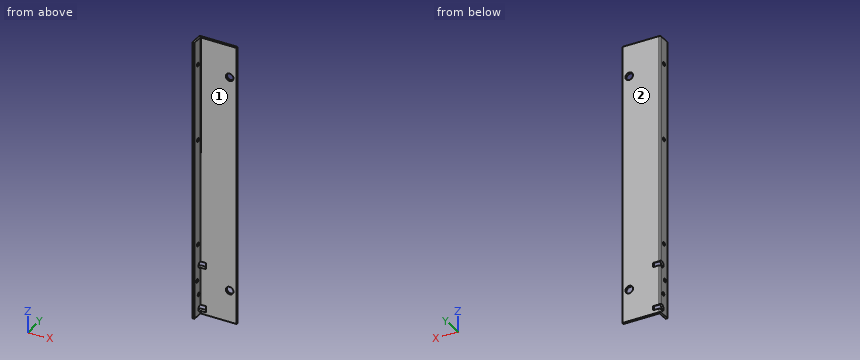
```python
from build123d import *

# Parameters (mm, degrees)
EXTRUDE_1_DEPTH     = 1100
SKETCH_2_R          = 15
CUT_EXTRUDE_1_DEPTH = 10
SKETCH_3_R          = 7
CUT_EXTRUDE_2_DEPTH = 10
SKETCH_4_R          = 12.5
CUT_EXTRUDE_3_DEPTH = 30
SKETCH_5_R          = 7
CUT_EXTRUDE_4_DEPTH = 10


with BuildPart() as part:
    # 草图1 → 凸台-拉伸1 (new body)
    with BuildSketch(Plane.XY):
        with BuildLine():
            Line((0, 0), (0, 45))
            ThreePointArc((0, 45), (1.464466094, 48.535533906), (5, 50))
            Line((5, 50), (150, 50))
            Line((150, 50), (150, 42))
            Line((150, 42), (10, 42))
            ThreePointArc((10, 42), (8.585786438, 41.414213562), (8, 40))
            Line((8, 40), (8, 0))
            Line((8, 0), (0, 0))
        make_face()
    extrude(amount=EXTRUDE_1_DEPTH)

    # 草图2 → 切除-拉伸1 (cut)
    with BuildSketch(Plane(origin=(0, 50, 0), x_dir=(1, 0, 0), z_dir=(0, 1, 0))):
        with Locations(Location((123, -975, 0), (0, 0, 270))):
            Circle(SKETCH_2_R)
        with Locations(Location((123, -125, 0), (0, 0, 270))):
            Circle(SKETCH_2_R)
    extrude(amount=-CUT_EXTRUDE_1_DEPTH, mode=Mode.SUBTRACT)

    # 草图3 → 切除-拉伸2 (cut)
    with BuildSketch(Plane.ZY):
        with Locations((283.54329503, 25.022549618)):
            Circle(SKETCH_3_R)
        with Locations((140.939449508, 19.704656779)):
            Circle(SKETCH_3_R)
        with Locations(Location((22.762519147, 40.542438099, 0), (0, 0, 355.555628173))):
            Circle(SKETCH_3_R)
        with Locations(Location((194.910597259, 40.650885608, 0), (0, 0, 354.6647218))):
            Circle(SKETCH_3_R)
        with Locations((81.850984328, 30.123547439)):
            Circle(SKETCH_3_R)
    extrude(amount=-CUT_EXTRUDE_2_DEPTH, mode=Mode.SUBTRACT)

    # 草图4 → 切除-拉伸3 (cut)
    with BuildSketch(Plane.ZY):
        with Locations((22.762519147, 40.542438099)):
            Circle(SKETCH_4_R)
        with Locations((194.910597259, 40.650885608)):
            Circle(SKETCH_4_R)
    extrude(amount=-CUT_EXTRUDE_3_DEPTH, mode=Mode.SUBTRACT)

    # 草图5 → 切除-拉伸4 (cut)
    with BuildSketch(Plane.ZY):
        with Locations((1000, 25.022549618)):
            Circle(SKETCH_5_R)
        with Locations((700, 25.022549618)):
            Circle(SKETCH_5_R)
    extrude(amount=-CUT_EXTRUDE_4_DEPTH, mode=Mode.SUBTRACT)


solid = part.part
```
Part model, mm, in its own coordinate system. Face numbers are marked on the shaded views. A direction names the side the tool comes from. Round coordinates to 2 decimals unless told otherwise and drop trailing zeros. Order: outer loops, then holes, each group sorted by start corner. A loop starts at its lowest first (then second) coordinate and runs counter-clockwise, first axis right, second up. Notation, with made-up numbers: M 68.5,-31 L 84.5,-31 A23 ccw 84.5,7 Z; hole C 83.25,-9 d7. An arc over 180 degrees is marked long. Answer in a Markdown table with one row per item. Add a question column.
Q1. Cut at D-D on x = 82.5. Give the cut face in (y, z), and give its area (3 significant figures).
Q2. Cut at B-B on x = 123. Give the cut face in (y, z), and give its area (3 significant figures).
Q3. 3-axis set-ups, long thin cutter, end or side, ignore diameter. For the marked faces 1 and 2: which of +Z, -Z, +X, -X, +Y, -Y reach the whole face in a straight line?
Q4. Cut at A-A on z = 975. Give the cut face in (x, y), and give its area (3 significant figures).
Q5. Wall check: L1, parallel to Z at x = 7, y = 23; L2, parallel to X at y = 44, z = 125; L3, parallel to Y at x = 108, z = 353. Give the ranges that are in metal, low to high. Write a range as from..to.
Q6. Pin check, flat tips, straight feed: pin 1 (12.5 mm diameter, centred on y = 19.7, z = 140.94, fed in from +X); pin 2 (10 mm diameter, centred on x = 89.5, z = 715.5, fed in from -Y); pin 3 (6.5 mm diameter, centred on y = 47, z = 18.5, fed in from -X); pin 4 (12 mm diameter, centred on y = 10, z = 685.5, fed in from +X). Stop position of each tip, or through.
Q7. Cut at C-C on z = 598. Give the cut face in (x, y).
Established:
| question | item | result |
|---|---|---|
| 1 | outline | M 42,0 L 50,0 L 50,1100 L 42,1100 Z |
| 1 | area | 8,800 mm2 |
| 2 | outline | M 42,0 L 50,0 L 50,110 L 42,110 Z; M 42,140 L 50,140 L 50,960 L 42,960 Z; M 42,990 L 50,990 L 50,1100 L 42,1100 Z |
| 2 | area | 8,320 mm2 |
| 3 | face 1 | +Z, -Z, +X, -Y |
| 3 | face 2 | +Z, -Z, +X, -X, +Y |
| 4 | outline | M 0,0 L 8,0 L 8,40 A2 cw 10,42 L 108,42 L 108,50 L 5,50 A5 ccw 0,45 Z; M 138,42 L 150,42 L 150,50 L 138,50 Z |
| 4 | area | 1,290 mm2 |
| 5 | L1 | z = 0..134.76, 147.12..276.84, 290.24..693.3, 706.7..993.3, 1006.7..1100 |
| 5 | L2 | x = 0..108, 138..150 |
| 5 | L3 | y = 42..50 |
| 6 | pin 1 | passes through |
| 6 | pin 2 | stops at y = 42 |
| 6 | pin 3 | stops at x = 30 |
| 6 | pin 4 | stops at x = 8 |
| 7 | outline | M 0,0 L 8,0 L 8,40 A2 cw 10,42 L 150,42 L 150,50 L 5,50 A5 ccw 0,45 Z |
